```python
from build123d import *

# Parameters (mm, degrees)
EXTRUDE_1_DEPTH     = 60
SKETCH_2_R          = 1.5
CUT_EXTRUDE_1_DEPTH = 10
SKETCH_3_R          = 2
CUT_EXTRUDE_2_DEPTH = 41


with BuildPart() as part:
    # 草图1 → 凸台-拉伸1 (new body)
    with BuildSketch(Plane(origin=(0, 0, 0), x_dir=(1, 0, 0), z_dir=(0, 1, 0))):
        with BuildLine():
            Line((-33.288662304, -40.97966402), (-33.288662304, -6.09314479))
            ThreePointArc((-33.288662304, -6.09314479), (-30.22599869, 2.989806272), (-22.288662304, 8.363687504))
            Line((-22.288662304, 8.363687504), (-22.288662304, 10.363687504))
            Line((-22.288662304, 10.363687504), (-14.288662304, 10.363687504))
            Line((-14.288662304, 10.363687504), (-14.288662304, 8.363687504))
            ThreePointArc((-14.288662304, 8.363687504), (-6.351325918, 2.989806272), (-3.288662304, -6.09314479))
            Line((-3.288662304, -6.09314479), (-3.288662304, -40.97966402))
            ThreePointArc((-3.288662304, -40.97966402), (-2.702875867, -42.393877582), (-1.288662304, -42.97966402))
            Line((-1.288662304, -42.97966402), (-0.288662304, -42.97966402))
            ThreePointArc((-0.288662304, -42.97966402), (1.125551258, -42.393877582), (1.711337696, -40.97966402))
            Line((1.711337696, -40.97966402), (1.711337696, 9.02033598))
            ThreePointArc((1.711337696, 9.02033598), (0.246871602, 12.555869886), (-3.288662304, 14.02033598))
            Line((-3.288662304, 14.02033598), (-33.288662304, 14.02033598))
            ThreePointArc((-33.288662304, 14.02033598), (-36.82419621, 12.555869886), (-38.288662304, 9.02033598))
            Line((-38.288662304, 9.02033598), (-38.288662304, -40.97966402))
            ThreePointArc((-38.288662304, -40.97966402), (-37.702875867, -42.393877582), (-36.288662304, -42.97966402))
            Line((-36.288662304, -42.97966402), (-35.288662304, -42.97966402))
            ThreePointArc((-35.288662304, -42.97966402), (-33.874448742, -42.393877582), (-33.288662304, -40.97966402))
        make_face()
    extrude(amount=EXTRUDE_1_DEPTH)

    # 草图2 → 切除-拉伸1 (cut)
    with BuildSketch(Plane.XY.offset(-10.363687504)):
        with Locations((-18.288662304, 50)):
            Circle(SKETCH_2_R)
        with Locations((-18.288662304, 30)):
            Circle(SKETCH_2_R)
        with Locations((-18.288662304, 10)):
            Circle(SKETCH_2_R)
    extrude(amount=-CUT_EXTRUDE_1_DEPTH, mode=Mode.SUBTRACT)

    # 草图3 → 切除-拉伸2 (cut, through all)
    with BuildSketch(Plane.ZY.offset(38.288662304)):
        with Locations((25.97966402, 50)):
            Circle(SKETCH_3_R)
        with Locations((25.97966402, 30)):
            Circle(SKETCH_3_R)
        with Locations((25.97966402, 10)):
            Circle(SKETCH_3_R)
    extrude(amount=-CUT_EXTRUDE_2_DEPTH, mode=Mode.SUBTRACT)


solid = part.part
```
Design review of the part built by this model. Coordinates are the model's own, in mm. A direction names the side the tool comes from. Coordinates: 2 decimals unless noted, no trailing zeros. Order: outer loops, then holes, each group sorted by start corner. A loop starts at its lowest first (then second) coordinate and runs counter-clockwise, first axis right, second up.
1) Clearance check with flat-ended pins moving along their axes: pin 1 (2 mm diameter, centred on x = -25, y = 27.5, fed in from +Z); pin 2 (6 mm diameter, centred on x = -12.5, y = 27, fed in from +Z); pin 3 (3 mm diameter, centred on x = -14.5, y = 37, fed in from +Z). State where each tip first meets the part, or that it passes through.
2) Take a section at C-C, the plane z = -3. Give the boundary of the cut face in (x, y).
3) Mouldability with a two-part tool opening along Z and no side actions: class faces 1 (the cylindrical face through (-30.31, 29.58, -2.88)), 2 (the cylindrical face through (-35.824, 48.783, 24.393)), 3 (the flat face through (-38.289, 30, 16)) as +Z half, -Z half, draft (parallel to the pull), parting line (faces both ways), or undercut.
4) Take a section at A-A, the plane y = 50. State how many separate pieces and enclosed holes the cut face has, and give its area (3 significant figures).
5) Take a section at D-D, the plane y = 19. Give the boundary of the cut face in (x, z).
6) Wall thickness on line 1 along X through (y, z) = (34.5, 16); line 2 along Z through (x, y) = (-15.5, 41); line 3 along Z through (x, y) = (-8.5, 33): over which ranges is each line inside the solid? List them lowest first.
7) For faces 4 (the cylindrical face through (-37.718, 29.58, 42.378)), 5 (the flat face through (-3.289, 30, 23)), list the 3-axis set-ups (+Z, -Z, +X, -X, +Y, -Y) from which the entire face can be reached by the end or side of a thin tool; tool diameter is ignored.
Returned:
1. pin 1: stops at z = -6.77
1. pin 2: stops at z = -6.06
1. pin 3: stops at z = -7.94
2. outline: (-38.29, 0) - (-30.22, 0) - (-30.22, 60) - (-38.29, 60) - close; (-6.36, 0) - (1.71, 0) - (1.71, 60) - (-6.36, 60) - close
3. face 1: +Z half
3. face 2: undercut
3. face 3: draft
4. separate pieces: 4
4. enclosed holes: 0
4. area: 742 mm2
5. outline: (-38.29, -9.02) arc R5 ccw to (-33.29, -14.02) - (-3.29, -14.02) arc R5 ccw to (1.71, -9.02) - (1.71, 40.98) arc R2 ccw to (-0.29, 42.98) - (-1.29, 42.98) arc R2 ccw to (-3.29, 40.98) - (-3.29, 6.09) arc R15 cw to (-14.29, -8.36) - (-14.29, -10.36) - (-22.29, -10.36) - (-22.29, -8.36) arc R15 cw to (-33.29, 6.09) - (-33.29, 40.98) arc R2 ccw to (-35.29, 42.98) - (-36.29, 42.98) arc R2 ccw to (-38.29, 40.98) - close
6. line 1: x = -38.29 to -33.29, -3.29 to 1.71
6. line 2: z = -14.02 to -10.36
6. line 3: z = -14.02 to -5.27
7. face 4: +Z, -X, +Y, -Y
7. face 5: +Z, +Y, -Y
